```python
from build123d import *

# Parameters (mm, degrees)
BOSS_EXTRUDE1_DEPTH = 15
CUT_EXTRUDE1_DEPTH  = 5
SKETCH4_R           = 0.75
CUT_EXTRUDE2_DEPTH  = 22.5


with BuildPart() as part:
    # Sketch1 → Boss-Extrude1 (new body)
    with BuildSketch(Plane(origin=(0, 0, 0), x_dir=(1, 0, 0), z_dir=(0, 1, 0))):
        Polygon((0, 0), (60, 0), (30, 30), align=None)
    extrude(amount=BOSS_EXTRUDE1_DEPTH)

    # Sketch3 → Cut-Extrude1 (cut)
    with BuildSketch(Plane(origin=(0, 15, 0), x_dir=(1, 0, 0), z_dir=(0, 1, 0))):
        Polygon((7.5, 7.5), (52.5, 7.5), (37.5, 22.5), (22.5, 22.5), align=None)
    extrude(amount=-CUT_EXTRUDE1_DEPTH, mode=Mode.SUBTRACT)

    # Sketch4 → Cut-Extrude2 (cut)
    with BuildSketch(Plane.XY):
        with Locations((20, 7.5)):
            Circle(SKETCH4_R)
        with Locations((40, 7.5)):
            Circle(SKETCH4_R)
    extrude(amount=-CUT_EXTRUDE2_DEPTH, mode=Mode.SUBTRACT)


solid = part.part
```
Check sheet for the modelled part. Datum: model origin and axes. Units: mm. A direction names the side the tool comes from. Round coordinates to 2 decimals unless told otherwise and drop trailing zeros. Order: outer loops, then holes, each group sorted by start corner. A loop starts at its lowest first (then second) coordinate and runs counter-clockwise, first axis right, second up. Notation, with made-up numbers: M -22,45.5 L -15,45.5 A25 ccw -15,77.5 Z; hole C 61,-17.5 d4. An arc over 180 degrees is marked long. Answer in a Markdown table with one row per item.
(1) Set-up check for faces 1 (the flat face through (30, 13, -7.5)), 2 (the flat face through (45, 6, -15)): record each of +Z, -Z, +X, -X, +Y, -Y from which the full face is reachable in a straight line by a thin tool's end or side.
Findings:
| item | result |
|---|---|
| face 1 | +X, -X, +Y |
| face 2 | -Z, +X, +Y, -Y |
(2) Section check A-A on y = 12.75. Record the boundary of the cut face in (x, z).
Findings:
| item | result |
|---|---|
| outline | M 0,0 L 7.5,-7.5 L 52.5,-7.5 L 60,0 Z; M 22.5,-22.5 L 30,-30 L 37.5,-22.5 Z |
(3) Section check C-C on z = -18. Record the boundary of the cut face in (x, y).
Findings:
| item | result |
|---|---|
| outline | M 18,0 L 42,0 L 42,10 L 18,10 Z; hole C 20,7.5 d1.5; hole C 40,7.5 d1.5 |
(4) Section check B-B on x = 40. Record the boundary of the cut face in (y, z), plus the area to 4 significant figures.
Findings:
| item | result |
|---|---|
| outline | M 0,-20 L 6.75,-20 L 6.75,0 L 0,0 Z; M 8.25,-20 L 10,-20 L 10,-7.5 L 15,-7.5 L 15,0 L 8.25,0 Z |
| area | 207.5 mm^2 |
(5) Material ranges on line 1 along X through (y, z) = (7.5, -7.5); line 2 along Y through (x, z) = (20, -11); line 3 along X through (y, z) = (7.5, -3.75), recorded low to high. Write a range as from..to.
Findings:
| item | result |
|---|---|
| line 1 | x = 7.5..19.25, 20.75..39.25, 40.75..52.5 |
| line 2 | y = 0..6.75, 8.25..10 |
| line 3 | x = 3.75..19.25, 20.75..39.25, 40.75..56.25 |
(6) Gauge pin test, flat ends, axial feed: pin 1 (1.5 mm diameter, centred on x = 43.5, y = 10, fed in from -Z); pin 2 (5 mm diameter, centred on x = 19.5, y = 3.5, fed in from -Z); pin 3 (4 mm diameter, centred on y = 13, z = -5.5, fed in from -X); pin 4 (0.9 mm diameter, centred on x = 40, y = 7.5, fed in from -Z). Record the tip position at first contact, or that the pin passes through.
Findings:
| item | result |
|---|---|
| pin 1 | stops at z = -17.25 |
| pin 2 | stops at z = -22 |
| pin 3 | stops at x = 3.5 |
| pin 4 | passes through |
(7) Section check D-D on y = 7.5. Record the boundary of the cut face in (x, z), plus the area to 3 significant figures.
Findings:
| item | result |
|---|---|
| outline | M 0,0 L 19.25,-19.25 L 19.25,0 Z; M 20.75,-20.75 L 30,-30 L 39.25,-20.75 L 39.25,0 L 20.75,0 Z; M 40.75,-19.25 L 60,0 L 40.75,0 Z |
| area | 840 mm^2 |
(8) Draft check along Y on faces 3 (the flat face through (30, 13, -22.5)), 4 (the flat face through (30, 10, -13)), 5 (the cylindrical face through (39.25, 7.53, -10.26)), 6 (the flat face through (30, 0, -12)). Enter one of: +Y half, -Y half, draft (parallel to the pull), parting line (faces both ways), or undercut.
Findings:
| item | result |
|---|---|
| face 3 | draft |
| face 4 | +Y half |
| face 5 | undercut |
| face 6 | -Y half |
